Part model, mm, in its own coordinate system. Round coordinates to 2 decimals unless told otherwise and drop trailing zeros. Loops run counter-clockwise (first coordinate to the right, second up) from the corner with the lowest first, then second, coordinate; pieces in that order, holes last.
(1) Flat gauge pins, fed straight in: pin 1 (1 mm diameter, centred on x = 4.5, z = -56, fed in from +Y); pin 2 (6 mm diameter, centred on x = -3, z = 58, fed in from +Y); pin 3 (0.7 mm diameter, centred on y = 5.5, z = 34.5, fed in from +X). Where does each tip first touch, or does it go through?
(2) Probe probe 1 along X at (y, z) = (0.5, 3); probe 2 along Y at (x, z) = (0.75, 69.5); probe 3 along X at (y, z) = (4.5, 19). List the from-to ranges inside material, lowest first.
(3) Cut at B-B on z = -39. List the corners of the cut face in (x, y), then the cut area to 3 significant figures.
(4) Cut at A-A on x = 0. List the corners of the cut face in (y, z), then the cut area to 3 significant figures.
from build123d import *

# Parameters (mm, degrees)
SKETCH1_R           = 6.35
EXTRUDE1_DEPTH      = 76.2
CHAMFER1_SIZE       = 0.9525
SKETCH3_W           = 3.175
SKETCH3_H           = 1.5875
EXTRUDE2_DEPTH      = 77.2
EXTRUDE2_DEPTH_BACK = 77.2


with BuildPart() as part:
    # Sketch1 → Extrude1 (new body, symmetric)
    with BuildSketch(Plane.XY):
        Circle(SKETCH1_R)
    extrude(amount=EXTRUDE1_DEPTH, both=True)

    # Chamfer1
    chamfer1_edges = [part.edges().sort_by_distance(p)[0] for p in [
        (-6.35, 0, -76.2),
        (-6.35, 0, 76.2),
    ]]
    chamfer(chamfer1_edges, length=CHAMFER1_SIZE)

    # Sketch3 → Extrude2 (cut, two sides)
    with BuildSketch(Plane.XY) as extrude2_sk:
        with Locations((0, 5.55625)):
            Rectangle(SKETCH3_W, SKETCH3_H)
    extrude(amount=EXTRUDE2_DEPTH, mode=Mode.SUBTRACT)
    extrude(extrude2_sk.sketch, amount=-EXTRUDE2_DEPTH_BACK, mode=Mode.SUBTRACT)


solid = part.part
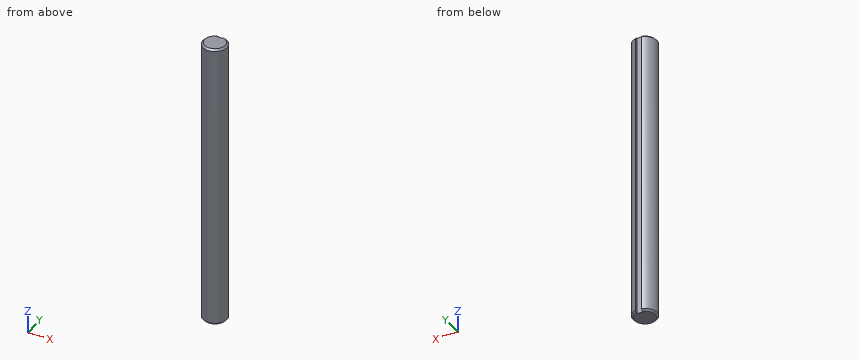
Final values:
1. pin 1: stops at y = 4.93
1. pin 2: stops at y = 6.15
1. pin 3: stops at x = 3.71
2. probe 1: x = -6.33 to 6.33
2. probe 2: y = -6.31 to 4.76
2. probe 3: x = -4.48 to 4.48
3. outline: (-1.59, 4.76) - (-1.59, 6.15) arc R6.35 ccw (long way) to (1.59, 6.15) - (1.59, 4.76) - close
3. area: 122 mm2
4. outline: (-6.35, -75.25) - (-5.4, -76.2) - (4.76, -76.2) - (4.76, 76.2) - (-5.4, 76.2) - (-6.35, 75.25) - close
4. area: 1,690 mm2
